For this review, take the finished solid that the model builds, in its own axes (mm). A direction names the side the tool comes from. Coordinates: 2 decimals unless noted, no trailing zeros. Order: outer loops, then holes, each group sorted by start corner. A loop starts at its lowest first (then second) coordinate and runs counter-clockwise, first axis right, second up.
from build123d import *

# Parameters (mm, degrees)
SKETCH1_R           = 11.43
SKETCH1_R_2         = 6.35
BOSS_EXTRUDE1_DEPTH = 19.939
WRAP1_START         = 6.056366153
WRAP1_DEPTH         = 6.35
WRAP1_2_DEPTH       = 1.13974359
WRAP1_START_2       = 8.417263589
WRAP1_3_DEPTH       = 1.13974359
WRAP1_START_3       = 11.266622564
WRAP1_4_DEPTH       = 1.139743589


# Read off the part's stored shape, not the designer's step: Wrap1
with BuildPart() as part:
    # Sketch1 → Boss-Extrude1 (new body)
    with BuildSketch(Plane.XY):
        Circle(SKETCH1_R)
        Circle(SKETCH1_R_2, mode=Mode.SUBTRACT)
    extrude(amount=BOSS_EXTRUDE1_DEPTH)

    # Wrap1 outline → Wrap1 (cut)
    with BuildSketch(Plane.XY.offset(WRAP1_START)):
        with BuildLine():
            Line((-0.598615526, 10.142349799), (-0.673442467, 11.410143524))
            ThreePointArc((-0.673442467, 11.410143524), (-1.24125177, 11.362402653), (-1.80597624, 11.286423252))
            Line((-1.80597624, 11.286423252), (-1.605312214, 10.032376224))
            ThreePointArc((-1.605312214, 10.032376224), (-1.103334907, 10.099913469), (-0.598615526, 10.142349799))
        make_face()
    extrude(amount=WRAP1_DEPTH, mode=Mode.SUBTRACT)

    # Wrap1 2 outline → Wrap1 2 (cut)
    with BuildSketch(Plane.XY.offset(WRAP1_START)):
        with BuildLine():
            Line((1.422558862, 10.059916813), (1.60037872, 11.317406415))
            ThreePointArc((1.60037872, 11.317406415), (0.465781866, 11.42050556), (-0.673442467, 11.410143524))
            Line((-0.673442467, 11.410143524), (-0.598615526, 10.142349799))
            ThreePointArc((-0.598615526, 10.142349799), (0.414028326, 10.151560498), (1.422558862, 10.059916813))
        make_face()
    extrude(amount=WRAP1_2_DEPTH, mode=Mode.SUBTRACT)

    # Wrap1 3 outline → Wrap1 3 (cut)
    with BuildSketch(Plane.XY.offset(WRAP1_START_2)):
        with BuildLine():
            Line((1.422558862, 10.059916813), (1.60037872, 11.317406415))
            ThreePointArc((1.60037872, 11.317406415), (0.465781866, 11.42050556), (-0.673442467, 11.410143524))
            Line((-0.673442467, 11.410143524), (-0.598615526, 10.142349799))
            ThreePointArc((-0.598615526, 10.142349799), (0.414028326, 10.151560498), (1.422558862, 10.059916813))
        make_face()
    extrude(amount=WRAP1_3_DEPTH, mode=Mode.SUBTRACT)

    # Wrap1 4 outline → Wrap1 4 (cut)
    with BuildSketch(Plane.XY.offset(WRAP1_START_3)):
        with BuildLine():
            Line((1.422558862, 10.059916813), (1.60037872, 11.317406415))
            ThreePointArc((1.60037872, 11.317406415), (0.465781866, 11.42050556), (-0.673442467, 11.410143524))
            Line((-0.673442467, 11.410143524), (-0.598615526, 10.142349799))
            ThreePointArc((-0.598615526, 10.142349799), (0.414028326, 10.151560498), (1.422558862, 10.059916813))
        make_face()
    extrude(amount=WRAP1_4_DEPTH, mode=Mode.SUBTRACT)


solid = part.part
1. Machinability: for faces 5 (the face through (0, 11, 12.406)), 6 (the face through (-0.636, 10.767, 7.798)), 7 (the face through (5, -5, 0)), which of the approach directions +Z, -Z, +X, -X, +Y, -Y give a long, thin tool a straight path to every point of the face, cutting with its end or side? Answer none if there is none.
Answer below:
face 5: +Y
face 6: none
face 7: -Z, +X, -X, +Y, -Y
2. Clearance check with flat-ended pins moving along their axes: pin 1 Ø2 at (y, z) = (4.5, 15) entering from +X; pin 2 Ø5 at (x, z) = (7, 9.5) entering from +Y; pin 3 Ø10 at (y, z) = (5.5, 16) entering from -X. State where each tip first meets the part, or that it passes through.
Answer below:
pin 1: stops at x = 10.88
pin 2: stops at y = 10.51
pin 3: stops at x = -11.42
3. To check wall thickness, follow L1, parallel to Y at x = 0, z = 11.5; L2, parallel to Y at x = 0, z = 5.75; L3, parallel to X at y = -4.25, z = 16.75. State the ranges of each line that lie inside material, in increasing order.
Answer below:
L1: y = -11.43 to -6.35, 6.35 to 10.16
L2: y = -11.43 to -6.35, 6.35 to 11.43
L3: x = -10.61 to -4.72, 4.72 to 10.61
4. The part is to be moulded in two halves that separate along Z. For faces 1 (the face through (0, 11, 7.196)), 2 (the face through (-1.38, -6.2, 9.83)), 3 (the face through (-0.636, 10.767, 10.4)), 4 (the face through (5, -5, 19.939)), say which applies: +Z half, -Z half, draft (parallel to the pull), parting line (faces both ways), or undercut.
Answer below:
face 1: undercut
face 2: draft
face 3: undercut
face 4: +Z half
5. Take a section at A-A, the plane y = 0. Give the boundary of the cut face in (x, z), plus the area to 3 significant figures.
Answer below:
outline: (-11.43, 0) - (-6.35, 0) - (-6.35, 19.94) - (-11.43, 19.94) - close; (6.35, 0) - (11.43, 0) - (11.43, 19.94) - (6.35, 19.94) - close
area: 203 mm2
6. Take a section at C-C, the plane z = 15.5. Give the boundary of the cut face in (x, y).
Answer below:
outline: circle Ø22.86 at (0, 0); hole circle Ø12.7 at (0, 0)
7. Take a section at B-B, the plane x = 0. Give the boundary of the cut face in (y, z).
Answer below:
outline: (-11.43, 0) - (-6.35, 0) - (-6.35, 19.94) - (-11.43, 19.94) - close; (6.35, 0) - (11.43, 0) - (11.43, 6.06) - (10.16, 6.06) - (10.16, 7.2) - (11.43, 7.2) - (11.43, 8.42) - (10.16, 8.42) - (10.16, 9.56) - (11.43, 9.56) - (11.43, 11.27) - (10.16, 11.27) - (10.16, 12.41) - (11.43, 12.41) - (11.43, 19.94) - (6.35, 19.94) - close
8. Take a section at D-D, the plane y = 3.5. Give the boundary of the cut face in (x, z).
Answer below:
outline: (-10.88, 0) - (-5.3, 0) - (-5.3, 19.94) - (-10.88, 19.94) - close; (5.3, 0) - (10.88, 0) - (10.88, 19.94) - (5.3, 19.94) - close
